For this review, take the finished solid that the model builds, in its own axes (mm). A direction names the side the tool comes from. Round coordinates to 2 decimals unless told otherwise and drop trailing zeros. Order: outer loops, then holes, each group sorted by start corner. A loop starts at its lowest first (then second) coordinate and runs counter-clockwise, first axis right, second up. Notation, with made-up numbers: M 34,60.5 L 86,60.5 A14 cw 86,79.5 Z; hole C 72,85.25 d7. An arc over 180 degrees is marked long. Use a Markdown table: item, result.
Autodesk Inventor part; units mm, degrees
ref_plane "YZ Plane" through (0, 0, 0) normal (1, 0, 0) x (0, 1, 0)
ref_plane "XZ Plane" through (0, 0, 0) normal (0, 1, 0) x (-1, 0, 0)
ref_plane "XY Plane" through (0, 0, 0) normal (0, 0, 1) x (1, 0, 0)
sketch "スケッチ1" plane through (0, 0, 0) normal (0, 1, 0) x (-1, 0, 0)
  line L0 (8.2, 28.6) -> (-8.2, 28.6)
  line L1 (-8.2, 28.6) -> (-8.2, -28.6)
  line L2 (-8.2, -28.6) -> (8.2, -28.6)
  line L3 (8.2, -28.6) -> (8.2, 28.6)
  line L4 (7, 26.6) -> (-7, 26.6)
  line L5 (-7, 26.6) -> (-7, -26.6)
  line L6 (-7, -26.6) -> (7, -26.6)
  line L7 (7, -26.6) -> (7, 26.6)
  point P0 (0, 0)
  point P1 (8.2, 0)
  point P2 (0, 28.6)
  point P3 (0, 26.6)
  point P4 (7, 0)
  dimension "d0" = 57.2
  dimension "d1" = 16.4
  dimension "d4" = 2
  dimension "d7" = 14
extrude "押し出し1" add sketch "スケッチ1" along normal blind 14
sketch "スケッチ2" plane through (-8.2, 0, 28.6) normal (0, 0, 1) x (1, 0, 0)
  circle A0 centre (8.2, 7) radius 7
  line L0 (0, 14) -> (16.4, 14)
  line L1 (0, 0) -> (16.4, 0)
  circle A1 centre (8.2, 7) radius 8.2
  line L2 (16.4, 0) -> (16.4, 14)
  line L3 (8.2, 7) -> (0, 14)
  line L4 (16.4, 14) -> (8.2, 7)
  line L5 (0, 0) -> (0, 14)
  point P0 (8.2, 0)
  point P1 (8.2, 0)
  point P2 (2.876, 11.5448)
  point P3 (1.9634, 12.324)
  point P4 (0, 7)
  point P5 (8.2, 0)
  point P6 (14.4366, 12.324)
  point P7 (13.524, 11.5448)
  point P8 (16.4, 7)
  point P9 (8.2, 14)
  dimension "d8" = 14
extrude "押し出し2" add sketch "スケッチ2" against normal up to surface (57.2 mm away) contours A0 L4 A1 L1 | L1 A1 L3 A0 | L1 L5 A1 | A1 L2 L1
extrude "押し出し3" cut sketch "スケッチ2" against normal through all contours A0 L0 A1 L4 | A0 L3 A1 L0 | L4 L2 A1 | A1 L0 L4 | A1 L3 L0 | A1 L5 L3
sketch "スケッチ3" plane through (0, 0, 0) normal (1, 0, 0) x (0, 1, 0)
  line L0 (0, 26.6) -> (11.5448, 26.6)
  line L1 (11.5448, -26.6) -> (11.5448, -26.6)
  line L2 (11.5448, -26.6) -> (0, -26.6)
  line L3 (0, -26.6) -> (11.5448, -26.6)
  line L4 (11.5448, 26.6) -> (11.5448, 26.6)
  line L5 (11.5448, 26.6) -> (0, 26.6)
  line L6 (0, 26.6) -> (11.5448, 26.6)
  line L7 (11.5448, 26.6) -> (14, 26.6)
  line L8 (14, -26.6) -> (11.5448, -26.6)
  line L9 (-2.8, 0) -> (16.8, 0)
  line L10 (14, 9) -> (6, 9)
  line L11 (6, 9) -> (6, -9)
  line L12 (6, -9) -> (14, -9)
  line L13 (14, 26.6) -> (6, 26.6)
  line L14 (6, 26.6) -> (6, 21.6)
  line L15 (6, 21.6) -> (14, 21.6)
  line L16 (14, 21.6) -> (14, 26.6)
  line L17 (14, -26.6) -> (6, -26.6)
  line L18 (6, -26.6) -> (6, -21.6)
  line L19 (6, -21.6) -> (14, -21.6)
  line L20 (14, -21.6) -> (14, -26.6)
  line L21 (14, 9) -> (14, -9)
  line L22 (0, 26.6) -> (0, -26.6)
  point P0 (0, 0)
  point P1 (12.7724, -26.6)
  point P2 (14, 0)
  point P3 (0, 0)
  dimension "d13" = 8
  dimension "d14" = 18
  dimension "d15" = 5
extrude "押し出し4" cut sketch "スケッチ3" along normal through all both and the other way through all
sketch "スケッチ4" plane through (0, 0, 0) normal (0, -1, 0) x (1, 0, 0)
  line L0 (-8.2, 28.6) -> (8.2, 28.6)
  line L1 (8.2, 28.6) -> (-8.2, 28.6)
  line L2 (-8.2, 28.6) -> (-8.2, -28.6)
  line L3 (-8.2, -28.6) -> (8.2, -28.6)
  line L4 (8.2, -28.6) -> (8.2, 28.6)
  point P0 (0, 0)
extrude "押し出し5" add sketch "スケッチ4" along normal blind 2
properties part number "AA_battery_box"
Q1. Add section A-A (x = 0). Write out the cut boundary in (y, z).
Determined:
| item | result |
|---|---|
| outline | M -2,-28.6 L 14,-28.6 L 14,-26.6 L 0,-26.6 L 0,26.6 L 14,26.6 L 14,28.6 L -2,28.6 Z |
Q2. Machinability: for faces 1 (the flat face through (8.2, 3, 0)), 2 (the flat face through (7, 9, 21.6)), 3 (the flat face through (0, 7, 26.6)), which of the approach directions +Z, -Z, +X, -X, +Y, -Y give a long, thin tool a straight path to every point of the face, cutting with its end or side? Answer none if there is none.
Determined:
| item | result |
|---|---|
| face 1 | +Z, -Z, +X, +Y, -Y |
| face 2 | +X, -X, +Y |
| face 3 | +Y |
Q3. Add section C-C (z = -14). Write out the cut boundary in (x, y), then the cut area to 3 significant figures.
Determined:
| item | result |
|---|---|
| outline | M -8.2,-2 L 8.2,-2 L 8.2,7 A8.2 ccw 6.24,12.32 L 5.32,11.54 A7 cw long -5.32,11.54 L -6.24,12.32 A8.2 ccw -8.2,7 Z |
| area | 83.5 mm^2 |
Q4. Clearance check with a flat-ended pin moving along its axis: pin 1 (1.4 mm diameter, centred on x = -7.5, z = -25, fed in from +Y). State where the tip first meets the part, or that it passes through.
Determined:
| item | result |
|---|---|
| pin 1 | stops at y = 6 |
Q5. Wall thickness on line 1 along Z through (x, y) = (-7, 8.5); line 2 along X through (y, z) = (7, -10); line 3 along Z through (x, y) = (5.75, 8): over which ranges is each line inside the solid? List them lowest first. Write a range as [from, to].
Determined:
| item | result |
|---|---|
| line 1 | z = [-28.6, -26.6], [-21.6, -9], [9, 21.6], [26.6, 28.6] |
| line 2 | x = [-8.2, -7], [7, 8.2] |
| line 3 | z = [-28.6, -26.6], [26.6, 28.6] |
Q6. Add section D-D (y = 2.75). Write out the cut boundary in (x, z), then the cut area to 3 significant figures.
Determined:
| item | result |
|---|---|
| outline | M -8.2,-28.6 L 8.2,-28.6 L 8.2,28.6 L -8.2,28.6 Z; hole M -5.56,-26.6 L 5.56,-26.6 L 5.56,26.6 L -5.56,26.6 Z |
| area | 346 mm^2 |
Q7. Draft analysis for pull direction Y (two halves, no side actions). For faces 4 (the flat face through (-7, 9, -9)), 5 (the cylindrical face through (-7.679, 9.875, -15.212)), 6 (the cylindrical face through (0, 0, 0)), state which applies: pulls with the +Y half, pulls with the -Y half, needs draft (parallel to the pull), parting line crosses it, or undercut.
Determined:
| item | result |
|---|---|
| face 4 | needs draft |
| face 5 | pulls with the +Y half |
| face 6 | undercut |
Q8. Add section B-B (y = 7.5). Write out the cut boundary in (x, z).
Determined:
| item | result |
|---|---|
| outline | M -8.18,-28.6 L 8.18,-28.6 L 8.18,-26.6 L -8.18,-26.6 Z; M -8.18,-21.6 L -6.98,-21.6 L -6.98,-9 L -8.18,-9 Z; M -8.18,9 L -6.98,9 L -6.98,21.6 L -8.18,21.6 Z; M -8.18,26.6 L 8.18,26.6 L 8.18,28.6 L -8.18,28.6 Z; M 6.98,-21.6 L 8.18,-21.6 L 8.18,-9 L 6.98,-9 Z; M 6.98,9 L 8.18,9 L 8.18,21.6 L 6.98,21.6 Z |
